For this review, take the finished solid that the model builds, in its own axes (mm). A direction names the side the tool comes from. Round coordinates to 2 decimals unless told otherwise and drop trailing zeros. Order: outer loops, then holes, each group sorted by start corner. A loop starts at its lowest first (then second) coordinate and runs counter-clockwise, first axis right, second up. Notation, with made-up numbers: (-39.75, 31) -> (-13.75, 31) arc R30 ccw to (-13.75, 66) -> close; hole circle Ø6 at (-34.5, 29.5). An arc over 180 degrees is marked (long way). Use a Markdown table: item, result. Add a question column.
1) Wall thickness on line 1 along X through (y, z) = (-18, -25); line 2 along Y through (x, z) = (40.5, -5); line 3 along Z through (x, y) = (378, -109.5): over which ranges is each line inside the solid? List them lowest first. Write a range as [from, to].
2) Machinability: for faces 1 (the face through (2, -48, -2)), 2 (the face through (0, -48, -2)), which of the approach directions +Z, -Z, +X, -X, +Y, -Y give a long, thin tool a straight path to every point of the face, cutting with its end or side? Answer none if there is none.
3) Consider section C-C (y = -87). State the section outline as (x, z) points, plus the area to 3 significant figures.
4) Clearance check with flat-ended pins moving along their axes: P1, Ø5, axis at x = 419, z = 46.5, coming from the +Y side; P2, Ø10, axis at x = 425.5, y = -73, coming from the +Z side; P3, Ø8, axis at x = 288, z = 85, coming from the +Y side. State where each tip first meets the part, or that it passes through.
5) Draft analysis for pull direction X (two halves, no side actions). For faces 3 (the face through (508, -48, -2)), 4 (the face through (250.44, -126.97, 2.79)), 5 (the face through (506, -48, -2)), 6 (the face through (250.47, -124.97, -2.75)), state which applies: pulls with the +X half, pulls with the -X half, needs draft (parallel to the pull), parting line crosses it, or undercut.
6) Consider section D-D (x = 280). State the section outline as (y, z) points, plus the area to 3 significant figures.
7) Consider section A-A (y = -29). State the section outline as (x, z) points, plus the area to 3 significant figures.
8) Consider section B-B (z = 79). State the section outline as (x, y) points, plus the area to 3 significant figures.
```python
from build123d import *

# Parameters (mm, degrees)
BOSS_EXTRUDE1_DEPTH = 508
BOSS_EXTRUDE2_START = -2
BOSS_EXTRUDE2_DEPTH = 2
LPATTERN1_COUNT     = 2
LPATTERN1_PITCH     = 506


with BuildPart() as part:
    # Sketch1 → Boss-Extrude1 (new body)
    with BuildSketch(Plane(origin=(0, 0, 0), x_dir=(0, 0, -1), z_dir=(1, 0, 0))):
        with BuildLine():
            Line((127, 0), (125, 0))
            ThreePointArc((125, 0), (0, -125), (-125, 0))
            Line((-125, 0), (-127, 0))
            ThreePointArc((-127, 0), (0, -127), (127, 0))
        make_face()
    extrude(amount=BOSS_EXTRUDE1_DEPTH)

    # Sketch2 → Boss-Extrude2 (add)
    with BuildSketch(Plane(origin=(508, 0, 0), x_dir=(0, 0, -1), z_dir=(1, 0, 0)).offset(BOSS_EXTRUDE2_START)):
        with BuildLine():
            Line((-125, 0), (125, 0))
            ThreePointArc((125, 0), (0, -125), (-125, 0))
        make_face()
    boss_extrude2 = extrude(amount=BOSS_EXTRUDE2_DEPTH)

    # LPattern1: Boss-Extrude2 ×2
    with Locations(*[(-i * LPATTERN1_PITCH, 0, 0) for i in range(1, LPATTERN1_COUNT)]):
        add(boss_extrude2)


solid = part.part
```
Results list:
| question | item | result |
|---|---|---|
| 1 | line 1 | [0, 2], [506, 508] |
| 1 | line 2 | [-126.9, -124.9] |
| 1 | line 3 | [-64.33, -60.29], [60.29, 64.33] |
| 2 | face 1 | +Y |
| 2 | face 2 | +Z, -Z, -X, +Y, -Y |
| 3 | outline | (0, -92.52) -> (508, -92.52) -> (508, 92.52) -> (0, 92.52) -> close; hole (2, -89.76) -> (506, -89.76) -> (506, 89.76) -> (2, 89.76) -> close |
| 3 | area | 3,530 mm2 |
| 4 | P1 | y = -115 |
| 4 | P2 | z = 107.26 |
| 4 | P3 | y = -87.77 |
| 5 | face 3 | pulls with the +X half |
| 5 | face 4 | needs draft |
| 5 | face 5 | undercut |
| 5 | face 6 | undercut |
| 6 | outline | (0, -127) -> (0, -125) arc R125 cw to (0, 125) -> (0, 127) arc R127 ccw to start |
| 6 | area | 792 mm2 |
| 7 | outline | (0, -123.64) -> (508, -123.64) -> (508, 123.64) -> (0, 123.64) -> close; hole (2, -121.59) -> (506, -121.59) -> (506, 121.59) -> (2, 121.59) -> close |
| 7 | area | 3,060 mm2 |
| 8 | outline | (0, -99.44) -> (508, -99.44) -> (508, 0) -> (506, 0) -> (506, -96.87) -> (2, -96.87) -> (2, 0) -> (0, 0) -> close |
| 8 | area | 1,690 mm2 |
